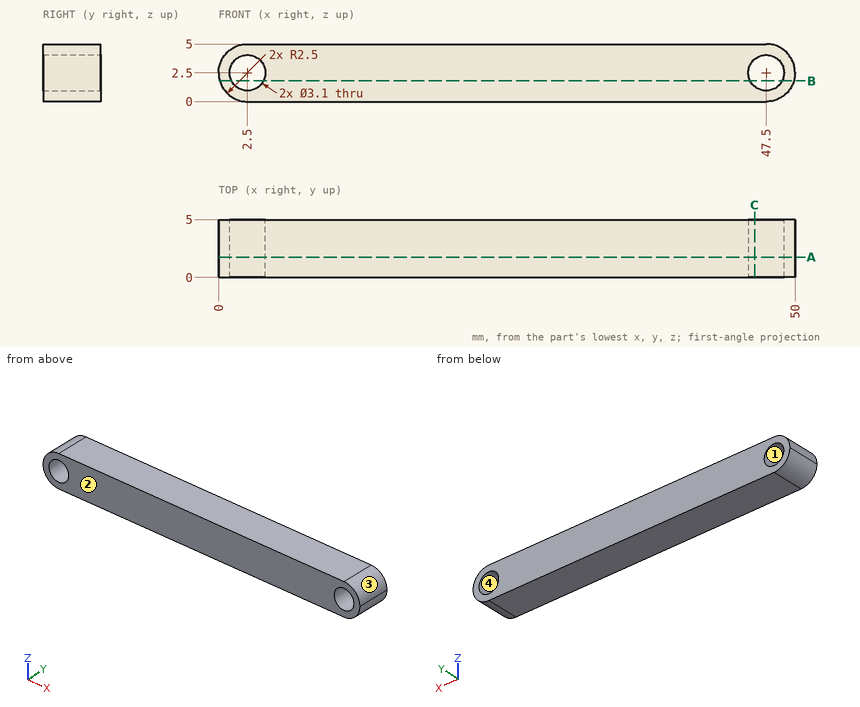
Verification items for this drawing (mm, ordinates from the low corner). Give positions to 0.01 mm unless a question says otherwise; leave off trailing zeros. Loops run counter-clockwise (first coordinate to the right, second up) from the corner with the lowest first, then second, coordinate; pieces in that order, holes last.
1. Material ranges on probe 1 along Z at (x, y) = (47.5, 2.4); probe 2 along X at (y, z) = (2.9, 1.15); probe 3 along X at (y, z) = (1.6, 2.35), recorded low to high.
Derived:
probe 1: z = 0 to 0.95, 4.05 to 5
probe 2: x = 0.4 to 1.74, 3.26 to 46.74, 48.26 to 49.6
probe 3: x = 0 to 0.96, 4.04 to 45.96, 49.04 to 50
2. Cross-section at C-C on x = 46.5. Record the cut outline in (y, z).
Derived:
outline: (0, 0) - (5, 0) - (5, 1.32) - (0, 1.32) - close; (0, 3.68) - (5, 3.68) - (5, 5) - (0, 5) - close
3. Release check for a two-part mould opening along Z. For the marked faces 1, 2, 3 and 4 record: +Z half, -Z half, draft (parallel to the pull), parting line (faces both ways), or undercut.
Derived:
face 1: undercut
face 2: draft
face 3: +Z half
face 4: undercut
4. Go/stop test with a flat-tipped pin: P1, Ø1.9, axis at x = 2.5, z = 2.5, coming from the -Y side. Record where the tip stops, or that it passes through.
Derived:
P1: passes through
5. Cross-section at B-B on z = 1.8. Record the cut outline in (x, y).
Derived:
outline: (0.1, 0) - (1.12, 0) - (1.12, 5) - (0.1, 5) - close; (3.88, 0) - (46.12, 0) - (46.12, 5) - (3.88, 5) - close; (48.88, 0) - (49.9, 0) - (49.9, 5) - (48.88, 5) - close
6. Cross-section at A-A on y = 1.75. Count the separate pieces of the cut face and the enclosed holes in it, and give its area (3 significant figures).
Derived:
separate pieces: 1
enclosed holes: 2
area: 230 mm2
